from build123d import *

# Parameters (mm, degrees)
F1_R     = 7
F2_DEPTH = 3


with BuildPart() as f2:
    # F1 (on Top) → F2 (new body)
    with BuildSketch(Plane.XY):
        with BuildLine():
            ThreePointArc((-96.278295, 114.530964), (-88.15041, 109.197131), (-85, 100))
            ThreePointArc((-85, 100), (-98.124327, 85.117734), (-114.530913, 96.278097))
            Line((-114.530913, 96.278097), (-89.998611, 0.5))
            Line((-89.998611, 0.5), (-0.5, 0.5))
            Line((-0.5, 0.5), (-0.5, 90))
            Line((-0.5, 90), (-96.278295, 114.530964))
        make_face()
        with BuildLine():
            ThreePointArc((-114.530913, 96.278097), (-98.124327, 85.117734), (-85, 100))
            ThreePointArc((-85, 100), (-88.15041, 109.197131), (-96.278295, 114.530964))
            ThreePointArc((-96.278295, 114.530964), (-110.606674, 110.60653), (-114.530913, 96.278097))
        make_face()
        with Locations((-100, 100)):
            Circle(F1_R, mode=Mode.SUBTRACT)
    extrude(amount=F2_DEPTH)


solid = f2.part
Design review of the part built by this model. Coordinates are the model's own, in mm. Round coordinates to 2 decimals unless told otherwise and drop trailing zeros. Write each loop counter-clockwise with the first axis right and the second up, starting at its lowest first coordinate (ties: lowest second). Pieces come first, ordered by that corner, then holes. Notation, with made-up numbers: M 12.25,-14.75 L 16.25,-14.75 A7 cw 16.25,-2.75 Z; hole C -37,-8 d7. An arc over 180 degrees is marked long. One line per item, written item: value. Start each with the question number.
1. Take a section at C-C on y = 100. State the section outline as (x, z) points.
2. Draft analysis for pull direction X (two halves, no side actions). For faces 1 (the face through (-59, 59, 3)), 2 (the face through (-105.16, 104.73, 1.48)), 3 (the face through (-110.45, 110.76, 1.48)), 4 (the face through (-0.5, 45, 1)), state which applies: pulls with the +X half, pulls with the -X half, needs draft (parallel to the pull), parting line crosses it, or undercut.
3. To check wall thickness, follow probe 1 along Y at (x, z) = (-86, 0.5); probe 2 along X at (y, z) = (38.5, 0.7); probe 3 along X at (y, z) = (26, 1.15). State the ranges of each line that lie inside material, in increasing order. Write a range as from..to.
4. Take a section at D-D on x = -17.5. State the section outline as (y, z) points.
5. Take a section at A-A on z = 2.2. State the section outline as (x, y) points.
6. Take a section at B-B on x = -100. State the section outline as (y, z) points, then the cut area to 3 significant figures.
7. Clearance check with a flat-ended pin moving along its axis: P1, Ø2, axis at x = -96, y = 21, coming from the -Z side. State where the tip first meets the part, or that it passes through.
Computed:
1. outline: M -115,0 L -107,0 L -107,3 L -115,3 Z; M -93,0 L -39.54,0 L -39.54,3 L -93,3 Z
2. face 1: needs draft
2. face 2: undercut
2. face 3: parting line crosses it
2. face 4: pulls with the +X half
3. probe 1: y = 0.5..111.9
3. probe 2: x = -99.73..-0.5
3. probe 3: x = -96.53..-0.5
4. outline: M 0.5,0 L 94.35,0 L 94.35,3 L 0.5,3 Z
5. outline: M -114.53,96.28 L -90,0.5 L -0.5,0.5 L -0.5,90 L -96.28,114.53 A15 ccw Z; hole C -100,100 d14
6. outline: M 39.55,0 L 93,0 L 93,3 L 39.55,3 Z; M 107,0 L 115,0 L 115,3 L 107,3 Z
6. area: 184 mm²
7. P1: stops at z = 0
